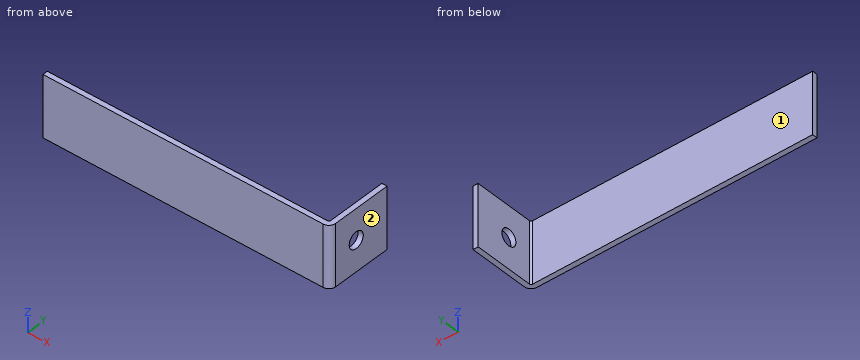
from build123d import *

# Parameters (mm, degrees)
SKETCH2_W                    = 177.8
SKETCH2_H                    = 38.1
BASE_FLANGE1_DEPTH           = 3.175
EDGE_FLANGE1_STRIP_W         = 14.7
EDGE_FLANGE1_STRIP_H         = 3.175
EDGE_FLANGE1_STRIP_CUT_DEPTH = 38.1
EDGE_FLANGE1_DEPTH           = 38.1
CUT_EXTRUDE1_REACH           = 184.749
SKETCH10_R                   = 5.08


# Sheet-metal steps are written as plain solids
with BuildPart() as part:
    # Sketch2 → Base-Flange1 (new body)
    with BuildSketch(Plane(origin=(0, 0, 0), x_dir=(1, 0, 0), z_dir=(0, 1, 0))):
        with Locations((88.9, 19.05)):
            Rectangle(SKETCH2_W, SKETCH2_H)
    extrude(amount=-BASE_FLANGE1_DEPTH)

    # Edge-Flange1 strip (across the edge) → Edge-Flange1 strip cut (cut)
    with BuildSketch(Plane(origin=(177.8, 0, 0), x_dir=(-1, 0, 0), z_dir=(0, 0, -1))):
        with Locations((-3.175, -1.5875)):
            Rectangle(EDGE_FLANGE1_STRIP_W, EDGE_FLANGE1_STRIP_H)
    extrude(amount=EDGE_FLANGE1_STRIP_CUT_DEPTH, mode=Mode.SUBTRACT)

    # Edge-Flange1 section (across the edge) → Edge-Flange1 (add)
    with BuildSketch(Plane(origin=(177.8, 0, 0), x_dir=(-1, 0, 0), z_dir=(0, 0, -1))):
        with BuildLine():
            Line((0, 1), (0, 38.1))
            Line((0, 38.1), (3.175, 38.1))
            Line((3.175, 38.1), (3.175, 1))
            ThreePointArc((3.175, 1), (3.467893219, 0.292893219), (4.175, 0))
            Line((4.175, 0), (4.175, -3.175))
            ThreePointArc((4.175, -3.175), (1.222829189, -1.952170811), (0, 1))
        make_face()
    extrude(amount=EDGE_FLANGE1_DEPTH)

    # Sketch10 → Cut-Extrude1 (cut, up to next)
    with BuildSketch(Plane.ZY.offset(-174.625), mode=Mode.PRIVATE) as cut_extrude1_sk1:
        with Locations(Location((-19.05, 15.875, 0), (0, 0, 270))):
            Circle(SKETCH10_R)
    cut_extrude1_tool1 = extrude(cut_extrude1_sk1.sketch, amount=-CUT_EXTRUDE1_REACH, mode=Mode.PRIVATE) & part.part
    add(cut_extrude1_tool1.solids().sort_by_distance((174.625, 15.875, -19.05))[0], mode=Mode.SUBTRACT)


solid = part.part
Geometry: final body of the model. Coordinates: model frame, mm. Face numbers are marked on the shaded views. A direction names the side the tool comes from. Round coordinates to 2 decimals unless told otherwise and drop trailing zeros. Order: outer loops, then holes, each group sorted by start corner. A loop starts at its lowest first (then second) coordinate and runs counter-clockwise, first axis right, second up. Notation, with made-up numbers: (-3.5, 30) -> (26.5, 30) arc R12 ccw to (26.5, 35) -> close; hole circle Ø1 at (-16.5, -14). An arc over 180 degrees is marked (long way). Put each result on its own line as item: value. Start each with the question number.
Q1. Line query: probe 1 along X at (y, z) = (18, -12) (3 decimals); probe 2 along Y at (x, z) = (105, -33.5) (3 decimals); probe 3 along Y at (x, z) = (176, -19). Output: solid intervals per line, ascending.
Q2. Reachability of the marked faces 1 and 2 from +Z, -Z, +X, -X, +Y, -Y: full face, straight path, thin tool, end or side. Return the list, or none.
Q3. Section B-B on y = 12.5. Return the cut outline in (x, z) (3 decimals), and give its area (3 significant figures).
Q4. Section C-C on z = -2.5. Return the cut outline in (x, y) (3 decimals).
Q5. First-contact query: pin 1 (12 mm diameter, centred on x = 158, z = -21.5, fed in from +Y); pin 2 (3 mm diameter, centred on y = 19, z = -21.5, fed in from -X) (3 decimals). Flat tips, straight axial feed; report the tip coordinate or a pass-through.
Q6. Section A-A on z = -19.05. Return the cut outline in (x, y) (3 decimals), and give its area (3 significant figures).
Q7. Section D-D on x = 141. Return the cut outline in (y, z) (3 decimals), and give its area (3 significant figures).
Ans:
1. probe 1: x = 174.625 to 177.8
1. probe 2: y = -3.175 to 0
1. probe 3: y = -2.43 to 10.8, 20.95 to 38.1
2. face 1: +Z, -Z, -X, +Y
2. face 2: +Z, -Z, +X, +Y, -Y
3. outline: (174.625, -38.1) -> (177.8, -38.1) -> (177.8, -22.847) -> (174.625, -22.847) -> close; (174.625, -15.253) -> (177.8, -15.253) -> (177.8, 0) -> (174.625, 0) -> close
3. area: 96.9 mm2
4. outline: (0, -3.175) -> (173.625, -3.175) arc R4.175 ccw to (177.8, 1) -> (177.8, 38.1) -> (174.625, 38.1) -> (174.625, 1) arc R1 cw to (173.625, 0) -> (0, 0) -> close
5. pin 1: stops at y = 0
5. pin 2: stops at x = 174.625
6. outline: (0, -3.175) -> (173.625, -3.175) arc R4.175 ccw to (177.8, 1) -> (177.8, 10.795) -> (174.625, 10.795) -> (174.625, 1) arc R1 cw to (173.625, 0) -> (0, 0) -> close; (174.625, 20.955) -> (177.8, 20.955) -> (177.8, 38.1) -> (174.625, 38.1) -> close
6. area: 650 mm2
7. outline: (-3.175, -38.1) -> (0, -38.1) -> (0, 0) -> (-3.175, 0) -> close
7. area: 121 mm2
